from build123d import *

# Parameters (mm, degrees)
SKETCH1_R           = 1
BOSS_EXTRUDE1_DEPTH = 4


with BuildPart() as part:
    # Sketch1 → Boss-Extrude1 (new body)
    with BuildSketch(Plane.XY):
        with BuildLine():
            ThreePointArc((5.156576759, 1.559717202), (3.671639417, 1.728041702), (2.228559137, 1.33959434))
            Line((2.228559137, 1.33959434), (-15.922809802, -7.447699535))
            ThreePointArc((-15.922809802, -7.447699535), (-19.613741884, -5.538880366), (-19.618658264, -1.383576999))
            Line((-19.618658264, -1.383576999), (-3.138918463, 8.524968964))
            ThreePointArc((-3.138918463, 8.524968964), (-1.594204388, 9.063420424), (0.036885671, 8.938453372))
            Line((0.036885671, 8.938453372), (13.428494888, 5.052778925))
            Line((13.428494888, 5.052778925), (19.826885957, 2.008227813))
            ThreePointArc((19.826885957, 2.008227813), (20.731162158, -0.159872308), (19.323277912, -2.040360419))
            Line((19.323277912, -2.040360419), (17.611370722, -2.303684453))
            Line((17.611370722, -2.303684453), (5.156576759, 1.559717202))
        make_face()
        with Locations((-16.832912189, -2.260702488)):
            Circle(SKETCH1_R, mode=Mode.SUBTRACT)
        with Locations((18.38085461, 0.132484859)):
            Circle(SKETCH1_R, mode=Mode.SUBTRACT)
    extrude(amount=BOSS_EXTRUDE1_DEPTH)


solid = part.part
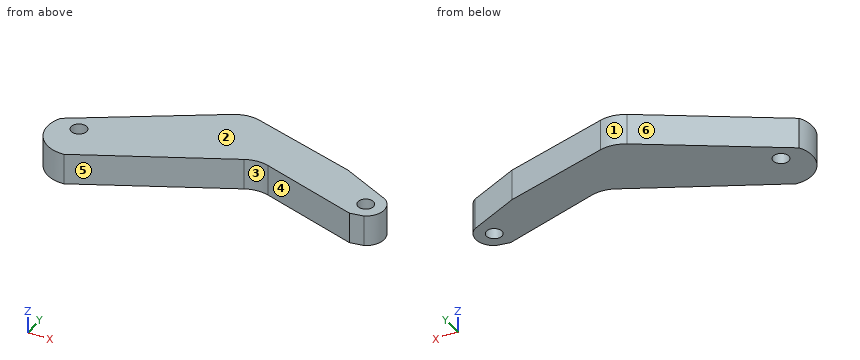
Here's how the part is built. I have some questions about the finished solid (model axes, mm). Face numbers are marked on the shaded views. A direction names the side the tool comes from. Give positions to 0.01 mm unless a question says otherwise; leave off trailing zeros. Write each loop counter-clockwise with the first axis right and the second up, starting at its lowest first coordinate (ties: lowest second). Pieces come first, ordered by that corner, then holes. Notation, with made-up numbers: (-20.75, 36.25) -> (11.25, 36.25) arc R20 ccw to (11.25, 73.25) -> close; hole circle Ø11 at (-18, -5.5). An arc over 180 degrees is marked (long way). Use one line per item in the form item = value. Start each with the question number.
1. Will these pins go through, and if not, where does the flat tip stop? pin 1 Ø1 at (x, z) = (-11, 1.5) entering from -Y; pin 2 Ø1 at (x, z) = (6.5, 3) entering from +Y; pin 3 Ø1 at (y, z) = (-1, 1) entering from +X.
2. If I drill on L1, parallel to Y at x = 18.5, z = 3.7; L2, parallel to X at y = 4.5, z = 2.55; L3, parallel to Y at x = 12, z = 1.75, over which ranges is the centre line in solid material (lowest first)?
3. On a 3-axis mill with a long thin cutter (end or side, diameter ignored), from which of +Z, -Z, +X, -X, +Y, -Y can I reach the whole of each face in a straight line? I mean the marked faces 5 and 6. Say none if no direction works.
4. Thinking about a two-plate mould opening in X: for the marked faces 1, 2, 3 and 4, which applies, +X half, -X half, draft (parallel to the pull), parting line (faces both ways), or undercut?
5. Imagine slicing it at A-A on z = 0.7. List the corners of the cut face in (x, y) for me.
6. Imagine slicing it at B-B on y = -4.75. List the corners of the cut face in (x, z) for me.
7. Imagine slicing it at C-C on x = -2. List the corners of the cut face in (y, z) for me, plus the area to 3 significant figures.
Entries:
q1.pin_1 = -5.31
q1.pin_2 = 7.21
q1.pin_3 = 20.66
q2.L1 = -2.17 to -0.86, 1.13 to 2.64
q2.L2 = -9.83 to 14.59
q2.L3 = -0.56 to 5.47
q3.face_5 = +Z, -Z, -Y
q3.face_6 = +Z, -Z, -X, +Y
q4.face_1 = parting line
q4.face_2 = draft
q4.face_3 = undercut
q4.face_4 = undercut
q5.outline = (-19.62, -1.38) arc R4 ccw to (-15.92, -7.45) -> (2.23, 1.34) arc R4 cw to (5.16, 1.56) -> (17.61, -2.3) -> (19.32, -2.04) arc R2.37 ccw to (19.83, 2.01) -> (13.43, 5.05) -> (0.04, 8.94) arc R4 ccw to (-3.14, 8.52) -> close; hole circle Ø2 at (-16.83, -2.26); hole circle Ø2 at (18.38, 0.13)
q6.outline = (-19.98, 0) -> (-10.35, 0) -> (-10.35, 4) -> (-19.98, 4) -> close
q7.outline = (-0.71, 0) -> (8.99, 0) -> (8.99, 4) -> (-0.71, 4) -> close
q7.area = 38.8 mm²
